from build123d import *

# Parameters (mm, degrees)
F0_W     = 71
F0_H     = 78.27916
F1_DEPTH = 25
F2_W     = 71
F2_H     = 78.27916
F3_DEPTH = 5


with BuildPart() as f1:
    # F0 (on Top) → F1 (new body)
    with BuildSketch(Plane.XY):
        Rectangle(F0_W, F0_H)
        Polygon((-30.5, -34.13958), (-30.5, -21.13958), (-25.5, -21.13958), (-25.5, -16.13958), (-30.5, -16.13958), (-30.5, 34.13958), (30.5, 34.13958), (30.5, -16.13958), (25.5, -16.13958), (25.5, -21.13958), (30.5, -21.13958), (30.5, -34.13958), align=None, mode=Mode.SUBTRACT)
    extrude(amount=F1_DEPTH)

    # F2 (on face) → F3 (join)
    with BuildSketch(Plane(origin=(0, 0, 0), x_dir=(1, 0, 0), z_dir=(0, 0, -1))):
        Rectangle(F2_W, F2_H)
        Polygon((-25.5, 34.13958), (25.5, 34.13958), (25.5, 16.13958), (30.5, 16.13958), (30.5, -34.13958), (-30.5, -34.13958), (-30.5, 16.13958), (-25.5, 16.13958), align=None, mode=Mode.SUBTRACT)
    extrude(amount=F3_DEPTH)


solid = f1.part
Can you work these out from the model? Positions are in its coordinate system, mm. A direction names the side the tool comes from. Coordinates: 2 decimals unless noted, no trailing zeros. Loops run counter-clockwise (first coordinate to the right, second up) from the corner with the lowest first, then second, coordinate; pieces in that order, holes last. Notation, with made-up numbers: M -23,-38 L 22,-38 A17 ccw 22,-6 Z; hole C 44,5 d1. An arc over 180 degrees is marked long. Return JSON: item names as keys, results as strings. Group by question number.
Item 1: Imagine slicing it at C-C (z = 8.75). Please give me the cut outline in (x, y).
Item 2: Imagine slicing it at B-B (x = 27). Please give me the cut outline in (y, z), and give its area (3 significant figures).
Item 3: If I drill on L1, parallel to X at y = -25.5, z = 6.25; L2, parallel to Y at x = -19, z = 3.5, over which ranges is the centre line in solid material (lowest first)? Write a range as from..to.
Item 4: On a 3-axis mill with a long thin cutter (end or side, diameter ignored), from which of +Z, -Z, +X, -X, +Y, -Y can I reach the whole of each face in a straight line? I mean faces 1 (the flat face through (-32, 1, 25)), 2 (the flat face through (-30.5, -28, 12)), 3 (the flat face through (0, 34.14, 10)). Say none if no direction works.
Item 5: Imagine slicing it at A-A (y = -20). Please give me the cut outline in (x, z).
Item 6: I'm going to push a flat-ended pin straight in: pin 1 Ø1.5 at (x, y) = (27.5, -25) entering from +Z. Where does the tip first touch, or does it pass through?
Item 7: Thinking about a two-plate mould opening in Y: for faces 4 (the flat face through (25.5, -20.5, 6.7)), 5 (the flat face through (0, 39.14, 10)), 6 (the flat face through (0, -39.14, 10)), which applies, released by +Y, released by -Y, zero draft, split by the parting line, or undercut?
Item 8: Imagine slicing it at D-D (y = 1). Please give me the cut outline in (x, z), and give its area (3 significant figures).
Verdict:
{
 "1": {"outline": "M -35.5,-39.14 L 35.5,-39.14 L 35.5,39.14 L -35.5,39.14 Z; hole M -30.5,-34.14 L 30.5,-34.14 L 30.5,-21.14 L 25.5,-21.14 L 25.5,-16.14 L 30.5,-16.14 L 30.5,34.14 L -30.5,34.14 L -30.5,-16.14 L -25.5,-16.14 L -25.5,-21.14 L -30.5,-21.14 Z"},
 "2": {"outline": "M -39.14,-5 L -16.14,-5 L -16.14,25 L -21.14,25 L -21.14,0 L -34.14,0 L -34.14,25 L -39.14,25 Z; M 34.14,-5 L 39.14,-5 L 39.14,25 L 34.14,25 Z", "area": "515 mm^2"},
 "3": {"L1": "x = -35.5..-30.5, 30.5..35.5", "L2": "y = -39.14..-34.14, 34.14..39.14"},
 "4": {"face 1": "+Z, +X, -X, +Y, -Y", "face 2": "+Z", "face 3": "+Z, -Z"},
 "5": {"outline": "M -35.5,-5 L -25.5,-5 L -25.5,25 L -35.5,25 Z; M 25.5,-5 L 35.5,-5 L 35.5,25 L 25.5,25 Z"},
 "6": {"pin 1": "stops at z = 0"},
 "7": {"face 4": "undercut", "face 5": "released by +Y", "face 6": "released by -Y"},
 "8": {"outline": "M -35.5,-5 L -30.5,-5 L -30.5,25 L -35.5,25 Z; M 30.5,-5 L 35.5,-5 L 35.5,25 L 30.5,25 Z", "area": "300 mm^2"}
}
